Autodesk Inventor part; units mm, degrees
ref_plane "YZ Plane" through (0, 0, 0) normal (1, 0, 0) x (0, 1, 0)
ref_plane "XZ Plane" through (0, 0, 0) normal (0, 1, 0) x (-1, 0, 0)
ref_plane "XY Plane" through (0, 0, 0) normal (0, 0, 1) x (1, 0, 0)
sketch "Эскиз" plane through (0, 0, 0) normal (1, 0, 0) x (0, 1, 0)
  circle A0 centre (0, 0) radius 3
  dimension "d1" = 6
extrude "Базовый элемент" add sketch "Эскиз" along normal blind 45
chamfer "Фаска1" distance 2 angle 30 1 edges at (0, -3, 0) measured on face at (15, 2.9612, -0.4812)
chamfer "Эскиз2" distance 2 angle 30 1 edges at (45, -3, 0) measured on face at (30.6667, 2.9903, -0.2414)
equation "\"d1\" = NND"
equation "\"d2\" = NLG"
equation "\"d8\" = PHH"
equation "\"d9\" = FAWI"
equation "\"d12\" = PHH"
equation "\"d4\" = PHH"
equation "\"d5\" = FAWI"
equation "\"d11\" = PHH"
equation "\"NND\" = 6"
equation "\"NLG\" = 45"
equation "\"PHH\" = 2"
equation "\"FAWI\" = 30deg"
equation "\"DIST1\" = 3.2"
equation "\"DIST2\" = DIST1"
equation "\"BOR1\" = 1.6"
equation "\"FAWI2\" = 30deg"
equation "\"BOR2\" = BOR1"
equation "\"PHH2\" = PHH"
properties part number "ISO 2340 - A - 6 x 45" material "Сталь"
Can you work these out from the model? Positions are in its coordinate system, mm. Give positions to 0.01 mm unless a question says otherwise; leave off trailing zeros. Order: outer loops, then holes, each group sorted by start corner. A loop starts at its lowest first (then second) coordinate and runs counter-clockwise, first axis right, second up. Notation, with made-up numbers: (48, -15) - (101, -15) arc R14 ccw to (101, 1) - close; hole circle Ø10 at (13.5, 63). An arc over 180 degrees is marked (long way). Use a Markdown table: item, result. Add a question column.
Q1. If we section it at A-A on z = 0: Write out the boundary of the cut face in (x, y), plus the area to 3 significant figures.
Q2. If we section it at C-C on x = 28: Write out the boundary of the cut face in (y, z).
Q3. Please list where these lines run through material, in increasing order: line 1 along Z through (x, y) = (9, -0.1); line 2 along X through (y, z) = (2.65, -0.25); line 3 along Z through (x, y) = (19.5, 0.9).
Q4. I'm going to push a flat-ended pin straight in: pin 1 (2 mm diameter, centred on x = 23.5, z = 1.5, fed in from -Y). Where does the tip first touch, or does it pass through?
Answers follow:
| question | item | result |
|---|---|---|
| 1 | outline | (0, -1.85) - (2, -3) - (43, -3) - (45, -1.85) - (45, 1.85) - (43, 3) - (2, 3) - (0, 1.85) - close |
| 1 | area | 265 mm^2 |
| 2 | outline | circle Ø6 at (0, 0) |
| 3 | line 1 | z = -3 to 3 |
| 3 | line 2 | x = 1.41 to 43.59 |
| 3 | line 3 | z = -2.86 to 2.86 |
| 4 | pin 1 | stops at y = -2.96 |
